```python
from build123d import *

# Parameters (mm, degrees)
SKETCH2_W               = 40.46
SKETCH2_H               = 55.31
BOSS_EXTRUDE1_DEPTH     = 2
SKETCH3_R               = 4
SKETCH3_R_2             = 1.5
BOSS_EXTRUDE2_DEPTH     = 4
FILLET1_R               = 2
SKETCH6_W               = 44.46
SKETCH6_H               = 59.31
SKETCH6_W_2             = 40.46
SKETCH6_H_2             = 55.31
BOSS_EXTRUDE3_DEPTH     = 17.5
SKETCH9_W               = 0.75
SKETCH9_H               = 5
CUT_EXTRUDE1_DEPTH      = 5
FILLET3_R               = 1
FILLET4_R               = 0.5
SKETCH12_W              = 44.46
SKETCH12_H              = 10
SKETCH12_W_2            = 40.46
SKETCH12_H_2            = 6
BOSS_EXTRUDE4_DEPTH     = 8
FILLET5_R               = 1
CUT_EXTRUDE2_DEPTH      = 10
CUT_EXTRUDE2_DEPTH_BACK = 8
SKETCH11_W              = 2
SKETCH11_H              = 2
SKETCH13_W              = 3.5
SKETCH13_H              = 2.5
CUT_EXTRUDE3_DEPTH      = 8
BOSS_EXTRUDE5_REACH     = 64.535
CUT_EXTRUDE4_DEPTH      = 48.832070201
CUT_EXTRUDE4_DEPTH_BACK = 48.832070201
SKETCH16_W              = 40.46
SKETCH16_H              = 6
SKETCH19_W              = 44.46
SKETCH19_H              = 10
SKETCH19_W_2            = 40.46
SKETCH19_H_2            = 6
BOSS_EXTRUDE7_DEPTH     = 9.5
SKETCH20_W              = 2
SKETCH20_H              = 2
CUT_EXTRUDE5_DEPTH      = 5


with BuildPart() as part:
    # Sketch2 → Boss-Extrude1 (new body)
    with BuildSketch(Plane(origin=(0, 0, 0), x_dir=(1, 0, 0), z_dir=(0, 1, 0))):
        with Locations((0, -2.5)):
            Rectangle(SKETCH2_W, SKETCH2_H)
    extrude(amount=BOSS_EXTRUDE1_DEPTH)

    # Sketch3 → Boss-Extrude2 (add)
    # profile 1 of 2: a face of its own
    with BuildSketch(Plane.XZ):
        with Locations(Location((-12.92, -17.845, 0), (0, 0, 90))):
            Circle(SKETCH3_R)
        with Locations(Location((-12.92, -17.845, 0), (0, 0, 270))):
            Circle(SKETCH3_R_2, mode=Mode.SUBTRACT)
    # profile 2 of 2: a face of its own
    with BuildSketch(Plane.XZ):
        with Locations(Location((11.5, -17.845, 0), (0, 0, 90))):
            Circle(SKETCH3_R)
        with Locations(Location((11.5, -17.845, 0), (0, 0, 270))):
            Circle(SKETCH3_R_2, mode=Mode.SUBTRACT)
    extrude(amount=BOSS_EXTRUDE2_DEPTH)

    # Fillet1
    fillet1_edges = [part.edges().sort_by_distance(p)[0] for p in [
        (-12.92, 0, -21.845),
        (11.5, 0, -21.845),
    ]]
    fillet(fillet1_edges, radius=FILLET1_R)

    # Sketch6 → Boss-Extrude3 (add)
    with BuildSketch(Plane(origin=(0, 2, 0), x_dir=(1, 0, 0), z_dir=(0, 1, 0))):
        with Locations((0, -2.5)):
            Rectangle(SKETCH6_W, SKETCH6_H)
        with Locations((0, -2.5)):
            Rectangle(SKETCH6_W_2, SKETCH6_H_2, mode=Mode.SUBTRACT)
    extrude(amount=-BOSS_EXTRUDE3_DEPTH)

    # Cut-Sweep1: sweep along a curve in space
    with BuildLine() as cut_sweep1_path:
        Line((-20.23, -15.5, -25.155), (-20.23, -15.5, 30.155))
    # Sketch9 → Cut-Sweep1 (sweep, cut)
    with BuildSketch(Plane(origin=(0, 0, 30.155), x_dir=(-1, 0, 0), z_dir=(0, 0, -1))):
        with Locations((20.605, -13)):
            Rectangle(SKETCH9_W, SKETCH9_H)
        with Locations((-20.605, -13)):
            Rectangle(SKETCH9_W, SKETCH9_H)
    sweep(path=cut_sweep1_path.line, mode=Mode.SUBTRACT)

    # Sketch10 → Cut-Extrude1 (cut)
    with BuildSketch(Plane.XZ.offset(15.5)):
        Polygon((-20.23, 30.155), (20.23, 30.155), (20.98, 30.155), (20.98, 30.905), (-20.98, 30.905), (-20.98, 30.155), align=None)
        Polygon((20.23, -25.155), (-20.23, -25.155), (-20.98, -25.155), (-20.98, -25.905), (20.98, -25.905), (20.98, -25.155), align=None)
    extrude(amount=-CUT_EXTRUDE1_DEPTH, mode=Mode.SUBTRACT)

    # Fillet3
    fillet3_edges = [part.edges().sort_by_distance(p)[0] for p in [
        (22.23, -6.75, 32.155),
        (22.23, -6.75, -27.155),
        (-22.23, -6.75, -27.155),
        (-22.23, -6.75, 32.155),
        (0, 2, -27.155),
        (22.23, 2, 2.5),
        (0, 2, 32.155),
        (-22.23, 2, 2.5),
        (-20.23, -5.25, 30.155),
        (-20.23, -5.25, -25.155),
        (20.23, -5.25, -25.155),
        (20.23, -5.25, 30.155),
        (0, 0, 30.155),
        (-20.23, 0, 2.5),
        (0, 0, -25.155),
        (20.23, 0, 2.5),
    ]]
    fillet(fillet3_edges, radius=FILLET3_R)

    # Fillet4
    fillet4_edges = [part.edges().sort_by_distance(p)[0] for p in [
        (20.98, -13, -25.905),
        (-20.98, -13, -25.905),
        (-20.98, -13, 30.905),
        (20.98, -13, 30.905),
    ]]
    fillet(fillet4_edges, radius=FILLET4_R)

    # Sketch12 → Boss-Extrude4 (add)
    # profile 1 of 2: a face of its own
    with BuildSketch(Plane(origin=(0, 2, 0), x_dir=(1, 0, 0), z_dir=(0, 1, 0))):
        with Locations((0, 31.155)):
            Rectangle(SKETCH12_W, SKETCH12_H)
        with Locations((0, 31.155)):
            Rectangle(SKETCH12_W_2, SKETCH12_H_2, mode=Mode.SUBTRACT)
    # profile 2 of 2: a face of its own
    with BuildSketch(Plane(origin=(0, 2, 0), x_dir=(1, 0, 0), z_dir=(0, 1, 0))):
        with Locations((0, -36.155)):
            Rectangle(SKETCH12_W, SKETCH12_H)
        with Locations((0, -36.155)):
            Rectangle(SKETCH12_W_2, SKETCH12_H_2, mode=Mode.SUBTRACT)
    extrude(amount=-BOSS_EXTRUDE4_DEPTH)

    # Fillet5
    fillet5_edges = [part.edges().sort_by_distance(p)[0] for p in [
        (-22.23, 2, 36.155),
        (-22.23, 2, -31.155),
        (22.23, 2, 36.155),
        (22.23, 2, -31.155),
    ]]
    fillet(fillet5_edges, radius=FILLET5_R)

    # Sketch11 → Cut-Extrude2 (cut, two sides: drawn at the far end of the back side and taken through both)
    with BuildSketch(Plane(origin=(0, 0, -27.155), x_dir=(-1, 0, 0), z_dir=(0, 0, -1)).offset(-CUT_EXTRUDE2_DEPTH_BACK)):
        with Locations((8.73, -8)):
            Rectangle(SKETCH11_W, SKETCH11_H)
    extrude(amount=CUT_EXTRUDE2_DEPTH + CUT_EXTRUDE2_DEPTH_BACK, mode=Mode.SUBTRACT)

    # Sketch13 → Cut-Extrude3 (cut)
    with BuildSketch(Plane(origin=(22.23, 0, 0), x_dir=(0, 0, -1), z_dir=(1, 0, 0))):
        with Locations((-1.595, -6.25)):
            Rectangle(SKETCH13_W, SKETCH13_H)
    extrude(amount=-CUT_EXTRUDE3_DEPTH, mode=Mode.SUBTRACT)

    # Boss-Extrude5: up to this face of the body (flat: up to its plane)
    boss_extrude5_end = Plane(part.part.faces().sort_by_distance((-22.23, -6.637443983, 2.5))[0])
    # Sketch14 → Boss-Extrude5 (add, up to the picked face)
    with BuildSketch(Plane(origin=(22.23, 0, 0), x_dir=(0, 0, -1), z_dir=(1, 0, 0)), mode=Mode.PRIVATE) as boss_extrude5_sk1:
        with BuildLine():
            Line((36.155, 4), (36.155, 1))
            Line((36.155, 1), (-41.155, 1))
            Line((-41.155, 1), (-41.155, 4))
            ThreePointArc((-41.155, 4), (-2.5, 1.964478359), (36.155, 4))
        make_face()
    boss_extrude5_tool1 = split(extrude(boss_extrude5_sk1.sketch, amount=-BOSS_EXTRUDE5_REACH, mode=Mode.PRIVATE), bisect_by=boss_extrude5_end, keep=Keep.BOTH, mode=Mode.PRIVATE)
    add(boss_extrude5_tool1.solids().sort_by(Axis((22.23, 1.933161, 2.5), (-1, 0, 0)))[0])

    # Sketch16 → Cut-Extrude4 (cut, two sides: drawn at the far end of the back side and taken through both)
    with BuildSketch(Plane.XZ.offset(6).offset(-CUT_EXTRUDE4_DEPTH_BACK)):
        with Locations((0, 36.155)):
            Rectangle(SKETCH16_W, SKETCH16_H)
        with Locations((0, -31.155)):
            Rectangle(SKETCH16_W, SKETCH16_H)
    extrude(amount=CUT_EXTRUDE4_DEPTH + CUT_EXTRUDE4_DEPTH_BACK, mode=Mode.SUBTRACT)

    # Sketch19 → Boss-Extrude7 (add)
    # profile 1 of 2: a face of its own
    with BuildSketch(Plane.XZ.offset(6)):
        with Locations((0, -31.155)):
            Rectangle(SKETCH19_W, SKETCH19_H)
        with Locations((0, -31.155)):
            Rectangle(SKETCH19_W_2, SKETCH19_H_2, mode=Mode.SUBTRACT)
    # profile 2 of 2: a face of its own
    with BuildSketch(Plane.XZ.offset(6)):
        with Locations((0, 36.155)):
            Rectangle(SKETCH19_W, SKETCH19_H)
        with Locations((0, 36.155)):
            Rectangle(SKETCH19_W_2, SKETCH19_H_2, mode=Mode.SUBTRACT)
    extrude(amount=BOSS_EXTRUDE7_DEPTH)

    # Sketch20 → Cut-Extrude5 (cut)
    with BuildSketch(Plane.XY.offset(-26.155)):
        with Locations((-8.73, -8)):
            Rectangle(SKETCH20_W, SKETCH20_H)
    extrude(amount=-CUT_EXTRUDE5_DEPTH, mode=Mode.SUBTRACT)


solid = part.part
```
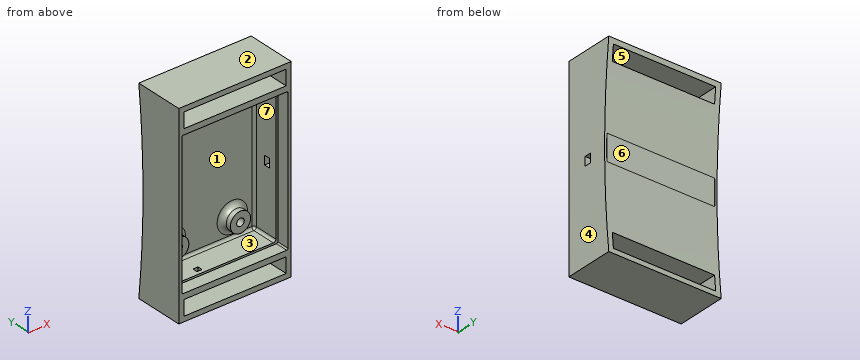
CAD build for the part. Positions are in the model's coordinates, mm. Face numbers are marked on the shaded views. A direction names the side the tool comes from. Round coordinates to 2 decimals unless told otherwise and drop trailing zeros. Order: outer loops, then holes, each group sorted by start corner. A loop starts at its lowest first (then second) coordinate and runs counter-clockwise, first axis right, second up. Notation, with made-up numbers: (77, 71.25) - (87, 71.25) arc R16 ccw to (87, 92.25) - close; hole circle Ø6 at (-2.75, -30.75). An arc over 180 degrees is marked (long way). Answer as CSV lines item,"result". Start each with the question number.
1. Drill centre lines: L1, parallel to Z at x = 6, y = -1.25 (3 decimals); L2, parallel to Z at x = -10.5, y = -11.75 (3 decimals); L3, parallel to Z at x = -4, y = 0.75 (3 decimals). Where is each one in solid material? Low to high. Write a range as [from, to].
2. Saw through at B-B, the plane y = 0.75. Write the cut outline in (x, z) (3 decimals).
3. Pull direction Z, two halves, no side cores. Call the marked faces 1, 2, 3 and 4: +Z half, -Z half, draft (parallel to the pull), parting line (faces both ways), or undercut.
4. Pin check, flat tips, straight feed: pin 1 (1.5 mm diameter, centred on x = 9.5, z = 21.5, fed in from -Y); pin 2 (10 mm diameter, centred on x = -16.5, z = 3, fed in from +Y); pin 3 (4 mm diameter, centred on x = 15, z = 28, fed in from +Y). Stop position of each tip, or through.
5. Tool access for the marked faces 5, 6 and 7: list every direction of +Z, -Z, +X, -X, +Y, -Y with a clear straight run to the whole face (end or side of a thin tool).
6. Saw through at D-D, the plane z = 14. Write the cut outline in (x, y).
7. Saw through at A-A, the plane x = -12.92. Count the separate pieces of the cut face and the enclosed holes in it, and give its area (3 significant figures).
8. Saw through at C-C, the plane z = 23. Write the cut outline in (x, y), and give its area (3 significant figures).
Model answer:
1,L1,"z = [-36.155, -34.155], [-28.155, -25.155], [30.155, 33.155], [39.155, 41.155]"
1,L2,"z = [-36.155, -34.155], [-28.155, -25.905], [30.905, 33.155], [39.155, 41.155]"
1,L3,"z = [-36.155, -34.155], [-28.155, 33.155], [39.155, 41.155]"
2,outline,"(-22.23, -36.155) - (22.23, -36.155) - (22.23, 41.155) - (-22.23, 41.155) - close; hole (-20.23, -34.155) - (20.23, -34.155) - (20.23, -28.155) - (-20.23, -28.155) - close; hole (-20.23, 33.155) - (20.23, 33.155) - (20.23, 39.155) - (-20.23, 39.155) - close"
3,face 1,"undercut"
3,face 2,"+Z half"
3,face 3,"undercut"
3,face 4,"draft"
4,pin 1,"stops at y = 0"
4,pin 2,"stops at y = 2.01"
4,pin 3,"stops at y = 2.99"
5,face 5,"+Y, -Y"
5,face 6,"+X, -X, +Y"
5,face 7,"-Y"
6,outline,"(-22.23, -15.5) - (-20.98, -15.5) - (-20.98, -10.5) - (-20.23, -10.5) - (-20.23, -1) arc R1 cw to (-19.23, 0) - (19.23, 0) arc R1 cw to (20.23, -1) - (20.23, -10.5) - (20.98, -10.5) - (20.98, -15.5) - (22.23, -15.5) - (22.23, 2.14) - (-22.23, 2.14) - close"
7,separate pieces,"3"
7,enclosed holes,"0"
7,area,"332 mm²"
8,outline,"(-22.23, -15.5) - (-20.98, -15.5) - (-20.98, -10.5) - (-20.23, -10.5) - (-20.23, -1) arc R1 cw to (-19.23, 0) - (19.23, 0) arc R1 cw to (20.23, -1) - (20.23, -10.5) - (20.98, -10.5) - (20.98, -15.5) - (22.23, -15.5) - (22.23, 2.54) - (-22.23, 2.54) - close"
8,area,"168 mm²"
